Here's how the part is built. I have some questions about the finished solid (model axes, mm). A direction names the side the tool comes from. Coordinates: 2 decimals unless noted, no trailing zeros. Write each loop counter-clockwise with the first axis right and the second up, starting at its lowest first coordinate (ties: lowest second). Pieces come first, ordered by that corner, then holes. Notation, with made-up numbers: M 14,18.5 L 60,18.5 A20 cw 60,25.5 Z; hole C 68.25,-6.75 d4. An arc over 180 degrees is marked long. Use a Markdown table: item, result.
Autodesk Inventor part; units mm, degrees
ref_plane "YZ Plane" through (0, 0, 0) normal (1, 0, 0) x (0, 1, 0)
ref_plane "XZ Plane" through (0, 0, 0) normal (0, 1, 0) x (-1, 0, 0)
ref_plane "XY Plane" through (0, 0, 0) normal (0, 0, 1) x (1, 0, 0)
sketch "Sketch1" plane through (0, 0, 0) normal (0, 0, 1) x (1, 0, 0)
  line L0 (0, 0) -> (38.1, 0)
  line L1 (38.1, 0) -> (38.1, 38.1)
  line L2 (38.1, 38.1) -> (0, 38.1)
  line L3 (0, 38.1) -> (0, 0)
  dimension "d0" = 38.1
  dimension "d1" = 38.1
extrude "Extrusion1" add sketch "Sketch1" along normal blind 3.175
sketch "Sketch2" plane through (0, 0, 3.175) normal (0, 0, 1) x (1, 0, 0)
  line L0 (0, 0) -> (38.1, 0)
  line L1 (38.1, 0) -> (38.1, 38.1)
  line L2 (0, 0) -> (38.1, 0)
  line L3 (38.1, 0) -> (38.1, 3.175)
  line L4 (38.1, 3.175) -> (0, 3.175)
  line L5 (0, 3.175) -> (0, 0)
  dimension "d4" = 3.175
extrude "Extrusion2" add sketch "Sketch2" along normal blind 38.1
sketch "Sketch3" plane through (0, 0, 0) normal (0, -1, 0) x (1, 0, 0)
  line L0 (0, 0) -> (38.1, 0)
  line L1 (0, 0) -> (0, 41.275)
  point P0 (25.4, 25.4)
  dimension "d7" = 25.4
  dimension "d8" = 25.4
hole "Hole1" at (25.4, 0, 25.4) direction (0, 1, 0) diameter 6.35 end through all
properties part number "CLB_064_ScissorOutsideLBraket"
1. Which directions (+Z, -Z, +X, -X, +Y, -Y) give clear straight access to the entire face, cutting with the end or side of a thin tool? Please do faces 1 (the face through (0, 2, 11)), 2 (the face through (19, 3.175, 22)).
Answers follow:
| item | result |
|---|---|
| face 1 | +Z, -Z, -X, +Y, -Y |
| face 2 | +Z, +X, -X, +Y |
2. Suppose I cut it at B-B on x = 25.4. Write out the boundary of the cut face in (y, z) (3 decimals), and give its area (3 significant figures).
Answers follow:
| item | result |
|---|---|
| outline | M 0,0 L 38.1,0 L 38.1,3.175 L 3.175,3.175 L 3.175,22.225 L 0,22.225 Z; M 0,28.575 L 3.175,28.575 L 3.175,41.275 L 0,41.275 Z |
| area | 222 mm2 |
3. We'd pull the mould along Z, two halves only. Please class faces 3 (the face through (19, 21, 3.175)), 4 (the face through (19, 0, 20)), 5 (the face through (24.45, 1.61, 22.37)), 6 (the face through (19, 19, 0)): +Z half, -Z half, draft (parallel to the pull), parting line (faces both ways), or undercut.
Answers follow:
| item | result |
|---|---|
| face 3 | +Z half |
| face 4 | draft |
| face 5 | undercut |
| face 6 | -Z half |
4. Will these pins go through, and if not, where does the flat tip stop? pin 1 Ø19 at (x, z) = (20.5, 27.5) entering from +Y (3 decimals); pin 2 Ø4 at (x, y) = (18, 7) entering from +Z (3 decimals).
Answers follow:
| item | result |
|---|---|
| pin 1 | stops at y = 3.175 |
| pin 2 | stops at z = 3.175 |
5. Suppose I cut it at A-A on z = 25.4. Write out the boundary of the cut face in (x, y) (3 decimals).
Answers follow:
| item | result |
|---|---|
| outline | M 0,0 L 22.225,0 L 22.225,3.175 L 0,3.175 Z; M 28.575,0 L 38.1,0 L 38.1,3.175 L 28.575,3.175 Z |
6. Suppose I cut it at D-D on y = 32.5. Write out the boundary of the cut face in (x, z) (3 decimals), and give its area (3 significant figures).
Answers follow:
| item | result |
|---|---|
| outline | M 0,0 L 38.1,0 L 38.1,3.175 L 0,3.175 Z |
| area | 121 mm2 |
7. Suppose I cut it at C-C on x = 36. Write out the boundary of the cut face in (y, z) (3 decimals), and give its area (3 significant figures).
Answers follow:
| item | result |
|---|---|
| outline | M 0,0 L 38.1,0 L 38.1,3.175 L 3.175,3.175 L 3.175,41.275 L 0,41.275 Z |
| area | 242 mm2 |
8. I need wall thicknesses on probe 1 along Z at (x, y) = (25.4, 1.6) (3 decimals); probe 2 along X at (y, z) = (1.95, 25.4) (3 decimals); probe 3 along Z at (x, y) = (9.5, 11) (3 decimals). Which ranges of each line are inside material? Lowest first, please.
Answers follow:
| item | result |
|---|---|
| probe 1 | z = 0 to 22.225, 28.575 to 41.275 |
| probe 2 | x = 0 to 22.225, 28.575 to 38.1 |
| probe 3 | z = 0 to 3.175 |
